Part model, mm, in its own coordinate system. A direction names the side the tool comes from. Round coordinates to 2 decimals unless told otherwise and drop trailing zeros. Loops run counter-clockwise (first coordinate to the right, second up) from the corner with the lowest first, then second, coordinate; pieces in that order, holes last.
1) Probe line 1 (X direction, y = 16, z = 6); line 2 (Y direction, x = 0, z = 2.35) (3 decimals); line 3 (Y direction, x = 3.5, z = 0.5) (3 decimals). List the from-to ranges inside material, lowest first.
2) Band-saw the part on A-A, the plane y = -6.5. Write the cut outline in (x, z).
3) Drop flat-ended pins along their axis: P1, Ø12, axis at x = 1, y = -13, coming from the +Z side; P2, Ø1.2, axis at x = -15, z = 6.5, coming from the +Y side; P3, Ø1.9, axis at y = 8, z = 6, coming from the +X side; P4, Ø2, axis at x = -21.52, y = 14.06, coming from the -Z side. Give the stop position or say it passes through.
4) 3-axis set-ups, long thin cutter, end or side, ignore diameter. For faces 1 (the flat face through (0, 16.525, 1)), 2 (the flat face through (11.3, 13, 6)), 3 (the cylindrical face through (-10.156, -4.358, 3.078)): which of +Z, -Z, +X, -X, +Y, -Y reach the whole face in a straight line?
5) Band-saw the part on B-B, the plane x = 1. Write the cut outline in (y, z) (3 decimals), then the cut area to 3 significant figures.
6) Band-saw the part on C-C, the plane y = 8. Write the cut outline in (x, z), then the cut area to 3 significant figures.
7) Mould opens along X. For faces 4 (the flat face through (-16.8, 9, 6)), 5 (the cylindrical face through (-11.91, -1.15, 5.92)), 6 (the cylindrical face through (12.64, 13.87, 3.5)) say: +X half, -X half, draft (parallel to the pull), parting line (faces both ways), or undercut.
from build123d import *

# Parameters (mm, degrees)
F0_W      = 66.9
F0_H      = 51.6
F1_DEPTH  = 1.5
F2_R      = 33.44999
F3_R      = 1.75
F5_DEPTH  = 10
F6_W      = 60
F6_H      = 1.5
F7_DEPTH  = 7
F8_W      = 28.5
F8_H      = 1.5
F9_DEPTH  = 13
F10_W     = 18
F10_H     = 1.5
F11_DEPTH = 31
F12_R     = 5
F13_R     = 1.75
F13_R_2   = 11.3
F15_DEPTH = 3.2
F16_R     = 10.7
F17_DEPTH = 3.2
F18_W     = 10
F18_H     = 8
F19_DEPTH = 5
F14_W     = 7.5
F14_H     = 7.5
F20_DEPTH = 25
F21_W     = 13.4
F21_H     = 4.7
F22_DEPTH = 5
F23_W     = 5.5
F23_H     = 20
F23_H_2   = 13
F24_DEPTH = 2.4
F25_R     = 1.75
F26_DEPTH = 25
F27_R     = 2.15
F28_R     = 0.3


# Not quite as in the source:
# - a fillet or chamfer is up to 0.001 mm smaller than in the source, because OpenCascade refuses the exact size
# - ends of sketch curves that miss each other by under 0.0002 mm in the source are joined


with BuildPart() as f1:
    # F0 (on Top) → F1 (new body)
    with BuildSketch(Plane.XY):
        Rectangle(F0_W, F0_H)
    extrude(amount=F1_DEPTH)

    # F2 (radius 33.45 in the source; OpenCascade refuses exactly that, so slightly less here)
    f2_edges = [f1.edges().sort_by_distance(p)[0] for p in [
        (-33.45, 25.8, 0.75),
        (33.45, 25.8, 0.75),
    ]]
    fillet(f2_edges, radius=F2_R)

    # F3 (on Top) → F5 (cut)
    with BuildSketch(Plane.XY):
        with Locations((-21.525, 14.0641658831)):
            Circle(F3_R)
        with Locations((-14.025, 12.8033463032)):
            Circle(F3_R)
        with Locations((21.525, 14.0641658831)):
            Circle(F3_R)
        with Locations((14.025, 12.8033463032)):
            Circle(F3_R)
    extrude(amount=F5_DEPTH, mode=Mode.SUBTRACT)

    # F6 (on face) → F7 (cut)
    with BuildSketch(Plane.YZ.offset(33.45)):
        with Locations((4.2, 0.75)):
            Rectangle(F6_W, F6_H)
    extrude(amount=-F7_DEPTH, mode=Mode.SUBTRACT)

    # F8 (on face) → F9 (cut)
    with BuildSketch(Plane.XZ.offset(25.8)):
        with Locations((-19.2, 0.75)):
            Rectangle(F8_W, F8_H)
    extrude(amount=-F9_DEPTH, mode=Mode.SUBTRACT)

    # F10 (on face) → F11 (cut)
    with BuildSketch(Plane.XZ.offset(25.8)):
        with Locations((17.45, 0.75)):
            Rectangle(F10_W, F10_H)
    extrude(amount=-F11_DEPTH, mode=Mode.SUBTRACT)

    # F12
    f12_edges = [f1.edges().sort_by_distance(p)[0] for p in [
        (8.45, 5.2, 0.75),
    ]]
    fillet(f12_edges, radius=F12_R)

    # F13 (on face) → F15 (join)
    with BuildSketch(Plane.XY.offset(1.5)):
        with BuildLine():
            ThreePointArc((8.45, 0.2), (9.9144660941, 3.7355339059), (13.45, 5.2))
            Line((13.45, 5.2), (26.45, 5.2))
            Line((26.45, 5.2), (26.45, 12.8268227403))
            ThreePointArc((26.45, 12.8268227403), (14.7301262522, 22.3820846236), (1e-05, 25.8))
            ThreePointArc((1e-05, 25.8), (-23.6527247596, 16.0027247596), (-33.45, -7.64999))
            Line((-33.45, -7.64999), (-33.45, -12.8))
            Line((-33.45, -12.8), (-4.95, -12.8))
            Line((-4.95, -12.8), (-4.95, -25.8))
            Line((-4.95, -25.8), (8.45, -25.8))
            Line((8.45, -25.8), (8.45, 0.2))
        make_face()
        with Locations((-14.025, 12.8033463032)):
            Circle(F13_R, mode=Mode.SUBTRACT)
        with Locations((-21.525, 14.0641658831)):
            Circle(F13_R, mode=Mode.SUBTRACT)
        with Locations((0, 12.775)):
            Circle(F13_R_2, mode=Mode.SUBTRACT)
        with Locations((14.025, 12.8033463032)):
            Circle(F13_R, mode=Mode.SUBTRACT)
        with Locations((21.525, 14.0641658831)):
            Circle(F13_R, mode=Mode.SUBTRACT)
    extrude(amount=F15_DEPTH)

    # F16 (on face) → F17 (cut)
    with BuildSketch(Plane.XY.offset(1.5)):
        with Locations((0, -7.725)):
            Circle(F16_R)
    extrude(amount=F17_DEPTH, mode=Mode.SUBTRACT)

    # F18 (on face) → F19 (cut)
    with BuildSketch(Plane.XY.offset(1.5)):
        Rectangle(F18_W, F18_H)
    extrude(amount=F19_DEPTH, mode=Mode.SUBTRACT)

    # F14 (on face) → F20 (cut)
    with BuildSketch(Plane(origin=(0, 0, 0), x_dir=(1, 0, 0), z_dir=(0, 0, -1))):
        with Locations((0, -12.775)):
            Rectangle(F14_W, F14_H)
        with Locations((0, 7.65)):
            Rectangle(F14_W, F14_H)
    extrude(amount=-F20_DEPTH, mode=Mode.SUBTRACT)

    # F21 (on face) → F22 (cut)
    with BuildSketch(Plane.XZ.offset(25.8)):
        with Locations((1.75, 2.35)):
            Rectangle(F21_W, F21_H)
    extrude(amount=-F22_DEPTH, mode=Mode.SUBTRACT)

    # F23 (on face) → F24 (join)
    with BuildSketch(Plane.XY.offset(4.7)):
        with Locations((-14.05, 8.2)):
            Rectangle(F23_W, F23_H)
        with Locations((14.05, 11.7)):
            Rectangle(F23_W, F23_H_2)
    extrude(amount=F24_DEPTH)

    # F25 (on face) → F26 (cut)
    with BuildSketch(Plane(origin=(0, 0, 0), x_dir=(1, 0, 0), z_dir=(0, 0, -1))):
        with Locations((14.025, -12.8033463032)):
            Circle(F25_R)
        with Locations((-14.025, -12.8033463032)):
            Circle(F25_R)
    extrude(amount=-F26_DEPTH, mode=Mode.SUBTRACT)

    # F27
    f27_edges = [f1.edges().sort_by_distance(p)[0] for p in [
        (11.3, 5.2, 5.9),
        (-11.3, -1.8, 5.9),
        (-16.8, -1.8, 5.9),
    ]]
    fillet(f27_edges, radius=F27_R)

    # F28
    f28_edges = [f1.edges().sort_by_distance(p)[0] for p in [
        (-9.419893, -12.8, 3.1),
        (5, 1.734915, 3.1),
        (8.45, -1.160893, 3.1),
        (8.45, -14.289107, 3.1),
        (-4.95, -17.211174, 3.1),
        (-5, 1.734915, 3.1),
    ]]
    fillet(f28_edges, radius=F28_R)


solid = f1.part
Reported:
1. line 1: x = -16.8 to -11.3, 11.3 to 16.8
1. line 2: y = -20.8 to -18.425, 24.075 to 25.8
1. line 3: y = -20.8 to -11.4, -3.9 to 9.025, 16.525 to 25.616
2. outline: (-33.43, 0) - (-3.75, 0) - (-3.75, 1.5) - (-10.63, 1.5) - (-10.63, 4.7) - (-33.43, 4.7) - close; (3.75, 0) - (8.45, 0) - (8.45, 1.5) - (3.75, 1.5) - close
3. P1: stops at z = 4.7
3. P2: stops at y = 18.2
3. P3: stops at x = 16.8
3. P4: passes through
4. face 1: +Z, -Z
4. face 2: +Z, +Y, -Y
4. face 3: +Z
5. outline: (-20.8, 0) - (-11.4, 0) - (-11.4, 1.5) - (-18.378, 1.5) - (-18.378, 4.7) - (-20.8, 4.7) - close; (-3.9, 0) - (9.025, 0) - (9.025, 1.5) - (-3.9, 1.5) - close; (16.525, 0) - (25.785, 0) - (25.785, 4.7) - (24.031, 4.7) - (24.031, 1.5) - (16.525, 1.5) - close
5. area: 60.7 mm2
6. outline: (-29.56, 0) - (26.45, 0) - (26.45, 4.7) - (16.8, 4.7) - (16.8, 7.1) - (11.3, 7.1) - (11.3, 4.7) - (10.24, 4.7) - (10.24, 1.5) - (-10.24, 1.5) - (-10.24, 4.7) - (-11.3, 4.7) - (-11.3, 7.1) - (-16.8, 7.1) - (-16.8, 4.7) - (-29.56, 4.7) - close
6. area: 224 mm2
7. face 4: -X half
7. face 5: +X half
7. face 6: undercut
